Verification items for the finished model (mm, model axes). Coordinates: 2 decimals unless noted, no trailing zeros. Order: outer loops, then holes, each group sorted by start corner. A loop starts at its lowest first (then second) coordinate and runs counter-clockwise, first axis right, second up. Notation, with made-up numbers: M 23,21.5 L 58,21.5 A31 ccw 58,55.5 Z; hole C 74.25,83 d10. An arc over 180 degrees is marked long. Return JSON: item names as keys, results as strings.
```python
from build123d import *

# Parameters (mm, degrees)
F1_DEPTH = 43.942


with BuildPart() as f1:
    # F0 (on Top) → F1 (new body, symmetric)
    with BuildSketch(Plane.XY):
        Polygon((-47.283915, -9.686464), (-37.366303, -30.550869), (-18.888521, -44.416438), (3.916393, -48.106737), (25.824109, -40.776361), (41.815833, -24.104613), (48.228053, -1.910788), (43.591808, 20.720775), (28.969205, 38.605458), (7.710106, 47.646096), (-15.315285, 45.771588), (-34.832129, 33.41136), (-46.369352, 13.396993), align=None)
    extrude(amount=F1_DEPTH, both=True)


solid = f1.part
```
Q1. Go/stop test with flat-tipped pins: pin 1 (1 mm diameter, centred on x = 15, z = 30.5, fed in from +Y); pin 2 (8 mm diameter, centred on y = -23.5, z = 33, fed in from +X); pin 3 (12 mm diameter, centred on y = 3.5, z = 20, fed in from +X). Record where each tip stops, or that it passes through.
Values:
{"pin 1": "y = 44.76", "pin 2": "x = 43.15", "pin 3": "x = 48.23"}
Q2. Cross-section at A-A, the plane z = -15. Record the boundary of the cut face in (x, y), and give its area (3 significant figures).
Values:
{"outline": "M -47.28,-9.69 L -37.37,-30.55 L -18.89,-44.42 L 3.92,-48.11 L 25.82,-40.78 L 41.82,-24.1 L 48.23,-1.91 L 43.59,20.72 L 28.97,38.61 L 7.71,47.65 L -15.32,45.77 L -34.83,33.41 L -46.37,13.4 Z", "area": "7,040 mm^2"}
Q3. Cross-section at B-B, the plane x = -30. Record the boundary of the cut face in (y, z), and give its area (3 significant figures).
Values:
{"outline": "M -36.08,-43.94 L 36.47,-43.94 L 36.47,43.94 L -36.08,43.94 Z", "area": "6,380 mm^2"}
Q4. Material ranges on line 1 along Y through (x, z) = (-40.5, 28.5); line 2 along Y through (x, z) = (7, -21.5); line 3 along X through (y, z) = (-3.5, -13.5), recorded low to high.
Values:
{"line 1": "-23.96 to 23.58", "line 2": "-47.07 to 47.59", "line 3": "-47.04 to 47.77"}
Q5. Cross-section at C-C, the plane y = 28. Record the boundary of the cut face in (x, z).
Values:
{"outline": "M -37.95,-43.94 L 37.64,-43.94 L 37.64,43.94 L -37.95,43.94 Z"}
